```python
from build123d import *

# Parameters (mm, degrees)
F1_DEPTH     = 80
F2_DEPTH     = 60
F3_DEPTH     = 30
F4_T4_ANGLE  = 321.2915133738
F4_S5_R      = 6.75
F4_T6_DEPTH  = 13
F4_T10_ANGLE = 330.397154177
F4_S11_R     = 6.3724602388
F4_T12_DEPTH = 12


# Not quite as in the source:
# - a fillet or chamfer that OpenCascade refuses, or shapes differently, is made with other operations: its cross-section is extruded or revolved along the edge and cut away or added


with BuildPart() as f1:
    # F0 (on Top) → F1 (new body)
    with BuildSketch(Plane.XY):
        with BuildLine():
            ThreePointArc((3.6719317522, -5.6638694553), (-6.7494746232, 0.0842158591), (3.8121072666, 5.5704881463))
            Line((3.8121072666, 5.5704881463), (3.8276649179, 6.1572300003))
            ThreePointArc((3.8276649179, 6.1572300003), (-7.2494177613, 0.091881022), (3.6703837587, -6.2522622357))
            Line((3.6703837587, -6.2522622357), (3.6719317522, -5.6638694553))
        make_face()
    extrude(amount=F1_DEPTH)

    # F0 (on Top) → F2 (join)
    with BuildSketch(Plane.XY):
        with BuildLine():
            Line((3.7829003883, 5.1256385395), (3.8121072666, 5.5704881463))
            ThreePointArc((3.8121072666, 5.5704881463), (-6.7494746232, 0.0842158591), (3.6719317522, -5.6638694553))
            Line((3.6719317522, -5.6638694553), (3.6728513037, -5.2038225677))
            ThreePointArc((3.6728513037, -5.2038225677), (-6.3764069894, 0.0685580429), (3.7829003883, 5.1256385395))
        make_face()
    extrude(amount=F2_DEPTH)

    # F0 (on Top) → F3 (join)
    with BuildSketch(Plane.XY):
        with BuildLine():
            Line((3.75369351, 4.6807889327), (3.7829003883, 5.1256385395))
            ThreePointArc((3.7829003883, 5.1256385395), (-6.3764069894, 0.0685580429), (3.6728513037, -5.2038225677))
            Line((3.6728513037, -5.2038225677), (3.6737708552, -4.7437756801))
            ThreePointArc((3.6737708552, -4.7437756801), (-5.9997842678, 0.0508796647), (3.75369351, 4.6807889327))
        make_face()
    extrude(amount=F3_DEPTH)

    # F4: chamfer of 1.5 on 2 edges, made by hand


with BuildPart() as f4_tool2:
    # F4_s3 → F4_t4 (revolve)
    with BuildSketch(Plane(origin=(-0.0002871576, -0.0007904765, 0), x_dir=(0, 0, 1), z_dir=(0.341440213, 0.9399034955, 0))):
        Polygon((60, 7.8681819087), (58.5, 6.3681819087), (60, 6.3681819087), align=None)
    revolve(axis=Axis((-0.004308375, 0.0006703174, 60), (0, 0, -1)), revolution_arc=F4_T4_ANGLE)

    # F4_s5 → F4_t6 (intersect, symmetric)
    with BuildSketch(Plane.XY.offset(59.2)):
        Circle(F4_S5_R)
    extrude(amount=F4_T6_DEPTH, both=True, mode=Mode.INTERSECT)


with BuildPart() as f1_1:
    add(f1.part)

    # F4_t1: cut F4_tool2
    add(f4_tool2.part, mode=Mode.SUBTRACT)


with BuildPart() as f4_tool8:
    # F4_s9 → F4_t10 (revolve)
    with BuildSketch(Plane(origin=(0, 0, 0), x_dir=(0, 0, 1), z_dir=(0.2636591374, 0.9646159128, 0))):
        Polygon((30, 7.5), (28.5, 6), (30, 6), align=None)
    revolve(axis=Axis((0, 0, 30), (0, 0, -1)), revolution_arc=F4_T10_ANGLE)

    # F4_s11 → F4_t12 (intersect, symmetric)
    with BuildSketch(Plane.XY.offset(29.2)):
        with Locations((-0.004308375, 0.0006703174)):
            Circle(F4_S11_R)
    extrude(amount=F4_T12_DEPTH, both=True, mode=Mode.INTERSECT)


with BuildPart() as f1_2:
    add(f1_1.part)

    # F4_t7: cut F4_tool8
    add(f4_tool8.part, mode=Mode.SUBTRACT)


solid = f1_2.part
```
Part model, mm, in its own coordinate system. Round coordinates to 2 decimals unless told otherwise and drop trailing zeros. Order: outer loops, then holes, each group sorted by start corner. A loop starts at its lowest first (then second) coordinate and runs counter-clockwise, first axis right, second up. Notation, with made-up numbers: M 71,54 L 91,54 A22 cw 91,91 Z; hole C 69,-14.5 d1. An arc over 180 degrees is marked long. Put each result on its own line as item: value. Start each with the question number.
1. Slice it at A-A on z = 19. List the corners of the cut face in (x, y), then the cut area to 3 significant figures.
2. Drop flat-ended pins along their axis: pin 1 (1 mm diameter, centred on x = -2, z = 66, fed in from +Y); pin 2 (5 mm diameter, centred on x = -3.5, y = -2, fed in from +Z); pin 3 (1 mm diameter, centred on x = -2, z = 37, fed in from -Y). Give the stop position or say it passes through.
3. Two-plate mould, pull along X, no slides. Class faces 1 (the face through (-6.521, -0.13, 58.645)), 2 (the face through (-6, 0, 14)), 3 (the face through (-6, 2, 0)), 4 (the face through (-7.244, 0.306, 39.44)): +X half, -X half, draft (parallel to the pull), parting line (faces both ways), or undercut.
4. Drill centre lines: probe 1 along Y at (x, z) = (0, 59.4); probe 2 along Y at (x, z) = (-3.5, 18.5); probe 3 along X at (y, z) = (0, 69). Where is each one in solid material? Low to high. Write a range as [from, to].
5. Slice it at B-B on z = 47. List the corners of the cut face in (x, y).
Findings:
1. outline: M 3.67,-6.25 L 3.67,-5.66 L 3.67,-4.74 A6 cw long 3.75,4.68 L 3.81,5.57 L 3.83,6.16 A7.25 ccw long Z
1. area: 35.9 mm2
2. pin 1: y = 7.09
2. pin 2: z = 58.66
2. pin 3: y = -7.09
3. face 1: undercut
3. face 2: undercut
3. face 3: draft
3. face 4: parting line
4. probe 1: [-7.25, -6.75], [6.75, 7.25]
4. probe 2: [-6.35, -4.87], [4.87, 6.35]
4. probe 3: [-7.25, -6.75]
5. outline: M 3.67,-6.25 L 3.67,-5.66 L 3.67,-5.2 A6.37 cw long 3.78,5.13 L 3.81,5.57 L 3.83,6.16 A7.25 ccw long Z
